CAD build for the part. Positions are in the model's coordinates, mm. Give positions to 0.01 mm unless a question says otherwise; leave off trailing zeros. Loops run counter-clockwise (first coordinate to the right, second up) from the corner with the lowest first, then second, coordinate; pieces in that order, holes last.
```python
from build123d import *

# Parameters (mm, degrees)
F0_W           = 24
F0_H           = 24
F0_R           = 2
F1_DEPTH       = 24
F6_D           = 4
F6_DEPTH       = 2
F6_TIP         = 1.2017212381
F7_D           = 4
F7_DEPTH       = 2
F7_TIP         = 1.2017212381
F8_D           = 4
F8_DEPTH       = 2
F8_TIP         = 1.2017212381
F9_D           = 4
F9_DEPTH       = 2
F9_TIP         = 1.2017212381
F9_ON_F5_D     = 4
F9_ON_F5_DEPTH = 2
F9_ON_F5_TIP   = 1.2017212381
F10_R          = 1


with BuildPart() as f1:
    # F0 (on Top) → F1 (new body)
    with BuildSketch(Plane.XY):
        Rectangle(F0_W, F0_H)
        with Locations((-6, -6)):
            Circle(F0_R, mode=Mode.SUBTRACT)
        with Locations((6, -6)):
            Circle(F0_R, mode=Mode.SUBTRACT)
        with Locations((-6, 6)):
            Circle(F0_R, mode=Mode.SUBTRACT)
        Circle(F0_R, mode=Mode.SUBTRACT)
        with Locations((6, 6)):
            Circle(F0_R, mode=Mode.SUBTRACT)
        with Locations((6, 6)):
            Circle(F0_R)
        with Locations((-6, 6)):
            Circle(F0_R)
        Circle(F0_R)
        with Locations((-6, -6)):
            Circle(F0_R)
        with Locations((6, -6)):
            Circle(F0_R)
    extrude(amount=F1_DEPTH)

    # F6
    with Locations(Plane.XZ.offset(12)):
        with Locations((-6, 18), (0, 12), (6, 6)):
            Hole(F6_D / 2, depth=F6_DEPTH)
            with Locations((0, 0, -(F6_DEPTH + F6_TIP / 2))):  # 118° drill point
                Cone(0, F6_D / 2, F6_TIP, mode=Mode.SUBTRACT)

    # F7
    with Locations(Plane(origin=(-12, 0, 0), x_dir=(0, -1, 0), z_dir=(-1, 0, 0))):
        with Locations((6, 19), (6, 12), (6, 5), (-6, 19), (-6, 12), (-6, 5)):
            Hole(F7_D / 2, depth=F7_DEPTH)
            with Locations((0, 0, -(F7_DEPTH + F7_TIP / 2))):  # 118° drill point
                Cone(0, F7_D / 2, F7_TIP, mode=Mode.SUBTRACT)

    # F8
    with Locations(Plane(origin=(0, 0, 0), x_dir=(1, 0, 0), z_dir=(0, 0, -1))):
        with Locations((-6, 6), (6, 6), (-6, -6), (6, -6), (0, 0)):
            Hole(F8_D / 2, depth=F8_DEPTH)
            with Locations((0, 0, -(F8_DEPTH + F8_TIP / 2))):  # 118° drill point
                Cone(0, F8_D / 2, F8_TIP, mode=Mode.SUBTRACT)

    # F9
    with Locations(Plane.YZ.offset(12)):
        with Locations((-6, 18), (6, 6)):
            Hole(F9_D / 2, depth=F9_DEPTH)
            with Locations((0, 0, -(F9_DEPTH + F9_TIP / 2))):  # 118° drill point
                Cone(0, F9_D / 2, F9_TIP, mode=Mode.SUBTRACT)

    # F9 on F5
    with Locations(Plane(origin=(0, 12, 0), x_dir=(-1, 0, 0), z_dir=(0, 1, 0))):
        with Locations((0, 12)):
            Hole(F9_ON_F5_D / 2, depth=F9_ON_F5_DEPTH)
            with Locations((0, 0, -(F9_ON_F5_DEPTH + F9_ON_F5_TIP / 2))):  # 118° drill point
                Cone(0, F9_ON_F5_D / 2, F9_ON_F5_TIP, mode=Mode.SUBTRACT)

    # F10
    f10_edges = [f1.edges().sort_by_distance(p)[0] for p in [
        (0, -12, 0),
        (-12, 0, 0),
        (-12, -12, 12),
        (12, 0, 0),
        (0, 12, 0),
        (12, -12, 12),
        (0, -12, 24),
        (-12, 0, 24),
        (-12, 12, 12),
        (0, 12, 24),
        (12, 12, 12),
        (12, 0, 24),
    ]]
    fillet(f10_edges, radius=F10_R)


solid = f1.part
```
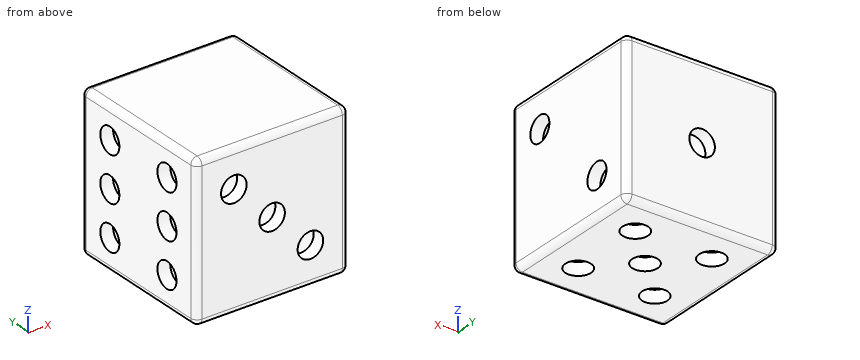
1. Saw through at A-A, the plane y = -9.5. List the corners of the cut face in (x, z), and give its area (3 significant figures).
Responses:
outline: (-12, 1) arc R1 ccw to (-11, 0) - (11, 0) arc R1 ccw to (12, 1) - (12, 23) arc R1 ccw to (11, 24) - (-11, 24) arc R1 ccw to (-12, 23) - close; hole circle Ø2.34 at (-6, 18); hole circle Ø2.34 at (0, 12); hole circle Ø2.34 at (6, 6)
area: 562 mm2
2. Probe line 1 along Z through (x, y) = (-10.35, -6); line 2 along Y through (x, z) = (6, 1.3); line 3 along Y through (x, z) = (-11.45, 5). List the from-to ranges inside material, lowest first.
Responses:
line 1: z = 0 to 3, 7 to 10, 14 to 17, 21 to 24
line 2: y = -12 to -8, -4 to 4, 8 to 12
line 3: y = -11.89 to -8, -4 to 4, 8 to 11.89
3. Drop flat-ended pins along their axis: pin 1 (2.5 mm diameter, centred on x = 6, y = 6, fed in from -Z); pin 2 (3.5 mm diameter, centred on y = -6, z = 19, fed in from +X); pin 3 (3.5 mm diameter, centred on y = -6, z = 5, fed in from -X); pin 4 (2.5 mm diameter, centred on x = 0, z = 12, fed in from +Y). Give the stop position or say it passes through.
Responses:
pin 1: stops at z = 2.45
pin 2: stops at x = 12
pin 3: stops at x = -9.85
pin 4: stops at y = 9.55
